The listing builds one solid part. Answer for the finished solid, in the listing's coordinates (mm). A direction names the side the tool comes from. Coordinates: 2 decimals unless noted, no trailing zeros. Loops run counter-clockwise (first coordinate to the right, second up) from the corner with the lowest first, then second, coordinate; pieces in that order, holes last. Notation, with made-up numbers: (22, 8) - (54, 8) arc R11 ccw to (54, 21) - close; hole circle Ø8 at (-2.5, 19.5). An arc over 180 degrees is marked (long way). Write each question's results on one line, items separated by ' | '. Start each with the question number.
(1) Find section C-C on z = 28.5. Determine the outline of the cut face in (x, y), then the cut area to 3 significant figures.
(2) Given pin 1 Ø3 at (y, z) = (0.5, 70) entering from -X; pin 2 Ø1.5 at (y, z) = (-4.5, 36) entering from -X; pin 3 Ø1 at (x, y) = (0, -0.5) entering from +Z, each flat-ended and moving along its own axis, determine where each tip first touches the part or whether it passes through.
(3) Find section D-D on x = -3.25. Determine the outline of the cut face in (y, z).
(4) Determine the mould class of faces 4 (the flat face through (-6, 1, 30.15)), 5 (the flat face through (0, 0, 67.005)), 6 (the cylindrical face through (-6.42, 0.28, 35.42)) for opening direction Y: released by +Y, released by -Y, zero draft, split by the parting line, or undercut.
(5) Consider line 1 (Y direction, x = 0, z = 74.25); line 2 (Z direction, x = 1, y = -0.25); line 3 (Z direction, x = -1.5, y = 5.5). Determine where each line is inside the solid, lowest interval first. Write a range as from..to.
(6) Find section A-A on y = 0. Determine the outline of the cut face in (x, z).
(7) For faces 1 (the cylindrical face through (-1.255, -5.653, 46.115)), 2 (the cylindrical face through (-1.255, -5.653, 28.514)), 3 (the flat face through (0, 0, 0)), determine the directions among +Z, -Z, +X, -X, +Y, -Y from which every point of the face is accessible in a straight line to the end or side of a thin tool.
from build123d import *

# Parameters (mm, degrees)
F0_R      = 5.5626
F1_DEPTH  = 26.924
F2_R      = 5.7912
F2_R_2    = 5.5626
F3_DEPTH  = 3.2258
F4_DEPTH  = 3.2258
F6_R      = 6.4262
F6_R_2    = 5.7912
F7_DEPTH  = 10.6934
F8_DEPTH  = 10.6934
F10_R     = 5.7912
F11_DEPTH = 10.6934
F12_R     = 5.5626
F13_DEPTH = 28.1686
F14_R     = 1.5875
F16_DEPTH = 12.7


with BuildPart() as f1:
    # F0 (on Top) → F1 (new body)
    with BuildSketch(Plane.XY):
        Circle(F0_R)
    extrude(amount=F1_DEPTH)

    # F2 (on face) → F3 (join)
    with BuildSketch(Plane.XY.offset(26.924)):
        Circle(F2_R)
        Circle(F2_R_2, mode=Mode.SUBTRACT)
    extrude(amount=F3_DEPTH)

    # F4 (add): a face of the model
    f4_faces = [f1.faces().sort_by_distance(p)[0] for p in [
        (0, 0, 26.924),
    ]]
    extrude(f4_faces, amount=F4_DEPTH)

    # F5: union 

    # F6 (on face) → F7 (join)
    with BuildSketch(Plane.XY.offset(30.1498)):
        Circle(F6_R)
        Circle(F6_R_2, mode=Mode.SUBTRACT)
    extrude(amount=F7_DEPTH)

    # F8 (add): a face of the model
    f8_faces = [f1.faces().sort_by_distance(p)[0] for p in [
        (0, 0, 30.1498),
    ]]
    extrude(f8_faces, amount=F8_DEPTH)

    # F9: union 

    # F10 (on face) → F11 (join)
    with BuildSketch(Plane.XY.offset(40.8432)):
        Circle(F10_R)
    extrude(amount=F11_DEPTH)

    # F12 (on face) → F13 (join)
    with BuildSketch(Plane.XY.offset(51.5366)):
        Circle(F12_R)
    extrude(amount=F13_DEPTH)

    # F14 (on face) → F16 (cut)
    with BuildSketch(Plane.XY.offset(79.7052)):
        Circle(F14_R)
    extrude(amount=-F16_DEPTH, mode=Mode.SUBTRACT)


solid = f1.part
Values:
1) outline: circle Ø11.58 at (0, 0) | area: 105 mm²
2) pin 1: stops at x = -5.56 | pin 2: stops at x = -5.22 | pin 3: stops at z = 67.01
3) outline: (-5.54, 30.15) - (-4.79, 30.15) - (-4.79, 26.92) - (-4.51, 26.92) - (-4.51, 0) - (4.51, 0) - (4.51, 26.92) - (4.79, 26.92) - (4.79, 30.15) - (5.54, 30.15) - (5.54, 40.84) - (4.79, 40.84) - (4.79, 51.54) - (4.51, 51.54) - (4.51, 79.71) - (-4.51, 79.71) - (-4.51, 51.54) - (-4.79, 51.54) - (-4.79, 40.84) - (-5.54, 40.84) - close
4) face 4: zero draft | face 5: undercut | face 6: split by the parting line
5) line 1: y = -5.56..-1.59, 1.59..5.56 | line 2: z = 0..67.01 | line 3: z = 26.92..51.54
6) outline: (-6.43, 30.15) - (-5.79, 30.15) - (-5.79, 26.92) - (-5.56, 26.92) - (-5.56, 0) - (5.56, 0) - (5.56, 26.92) - (5.79, 26.92) - (5.79, 30.15) - (6.43, 30.15) - (6.43, 40.84) - (5.79, 40.84) - (5.79, 51.54) - (5.56, 51.54) - (5.56, 79.71) - (1.59, 79.71) - (1.59, 67.01) - (-1.59, 67.01) - (-1.59, 79.71) - (-5.56, 79.71) - (-5.56, 51.54) - (-5.79, 51.54) - (-5.79, 40.84) - (-6.43, 40.84) - close
7) face 1: +Z | face 2: -Z | face 3: -Z, +X, -X, +Y, -Y
